Model file for the job. Use its own axes, mm. Face numbers are marked on the shaded views. A direction names the side the tool comes from. Coordinates: 2 decimals unless noted, no trailing zeros. Order: outer loops, then holes, each group sorted by start corner. A loop starts at its lowest first (then second) coordinate and runs counter-clockwise, first axis right, second up.
from build123d import *

# Parameters (mm, degrees)
SKETCH1_W           = 237.666601654
SKETCH1_H           = 144.870829151
BOSS_EXTRUDE1_DEPTH = 6.35
SKETCH6_R           = 4.7625
CUT_EXTRUDE1_DEPTH  = 279.412092375
BOSS_EXTRUDE2_DEPTH = 31.75
SKETCH8_R           = 3.5814
CUT_EXTRUDE2_DEPTH  = 165.026783357
FILLET1_R           = 3.81


with BuildPart() as part:
    # Sketch1 → Boss-Extrude1 (new body)
    with BuildSketch(Plane.XY):
        with Locations((118.833300827, 72.435414576)):
            Rectangle(SKETCH1_W, SKETCH1_H)
    extrude(amount=BOSS_EXTRUDE1_DEPTH)

    # Sketch6 → Cut-Extrude1 (cut, through all)
    with BuildSketch(Plane(origin=(0, 0, 0), x_dir=(-1, 0, 0), z_dir=(0, 0, -1))):
        with Locations((-216.35760516, 91.973324775)):
            Circle(SKETCH6_R)
        with Locations(Location((-118.912497493, 20.833508274, 0), (0, 0, 180))):
            Circle(SKETCH6_R)
        with BuildLine():
            Line((-237.666601654, 102.132216913), (-216.358133389, 102.133324761))
            ThreePointArc((-216.358133389, 102.133324761), (-208.163913134, 97.980737777), (-206.668218378, 88.91695703))
            Line((-206.668218378, 88.91695703), (-209.863652574, 78.786697699))
            ThreePointArc((-209.863652574, 78.786697699), (-210.516155402, 72.927274811), (-208.895904566, 67.258643251))
            Line((-208.895904566, 67.258643251), (-194.461394125, 39.056254914))
            ThreePointArc((-194.461394125, 39.056254914), (-186.82764399, 30.114000126), (-175.984822796, 25.567431049))
            Line((-175.984822796, 25.567431049), (-144.725556293, 20.41107019))
            ThreePointArc((-144.725556293, 20.41107019), (-138.832778099, 20.5948137), (-133.450682209, 23.001396414))
            Line((-133.450682209, 23.001396414), (-124.775487304, 29.13115556))
            ThreePointArc((-124.775487304, 29.13115556), (-114.240366099, 29.855525136), (-108.752497493, 20.833508274))
            Line((-108.752497493, 20.833508274), (-108.752497493, 0))
            Line((-108.752497493, 0), (33.78855799, -29.414686869))
            Line((33.78855799, -29.414686869), (48.645656143, 190.527142522))
            Line((48.645656143, 190.527142522), (-347.111633803, 192.661310616))
            Line((-347.111633803, 192.661310616), (-237.666601654, 102.132216913))
        make_face()
    extrude(amount=-CUT_EXTRUDE1_DEPTH, mode=Mode.SUBTRACT)

    # Sketch7 → Boss-Extrude2 (add)
    with BuildSketch(Plane.XY.offset(6.35)):
        Polygon((231.316601654, 102.132547055), (237.666601654, 102.132216913), (237.666601654, 0), (231.316601654, 0), align=None)
    extrude(amount=BOSS_EXTRUDE2_DEPTH)

    # Sketch8 → Cut-Extrude2 (cut, through all)
    with BuildSketch(Plane.ZY.offset(-231.316601654)):
        with Locations((23.289062999, 76.03064494)):
            Circle(SKETCH8_R)
        with Locations((23.289062999, 28.982263142)):
            Circle(SKETCH8_R)
    extrude(amount=-CUT_EXTRUDE2_DEPTH, mode=Mode.SUBTRACT)

    # Fillet1
    fillet1_edges = [part.edges().sort_by_distance(p)[0] for p in [
        (108.752497493, 0, 3.175),
        (231.316601654, 51.066273528, 6.35),
        (234.491601654, 0, 38.1),
        (234.491601654, 102.132381984, 38.1),
    ]]
    fillet(fillet1_edges, radius=FILLET1_R)


solid = part.part
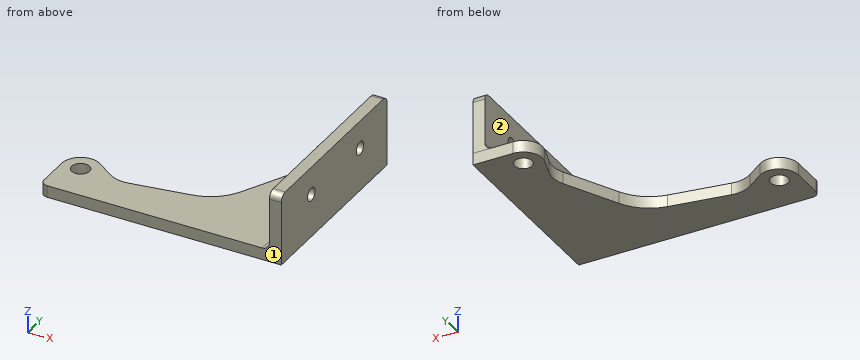
Q1. Cut at A-A, the plane x = 219. List the corners of the cut face in (y, z), plus the area to 3 significant figures.
Established:
outline: (0, 0) - (88.01, 0) - (88.01, 6.35) - (0, 6.35) - close; (95.94, 0) - (102.13, 0) - (102.13, 6.35) - (95.94, 6.35) - close
area: 598 mm2
Q2. Cut at C-C, the plane y = 84.5. List the corners of the cut face in (x, z), plus the area to 3 significant figures.
Established:
outline: (208.06, 0) - (237.67, 0) - (237.67, 38.1) - (231.32, 38.1) - (231.32, 10.16) arc R3.81 cw to (227.51, 6.35) - (208.06, 6.35) - close
area: 393 mm2
Q3. Cut at B-B, the plane z = 3.5. List the corners of the cut face in (x, y) (1 decimal).
Established:
outline: (108.8, 3.8) arc R3.8 ccw to (112.6, 0) - (237.7, 0) - (237.7, 102.1) - (216.4, 102.1) arc R10.2 ccw to (206.7, 88.9) - (209.9, 78.8) arc R15.2 cw to (208.9, 67.3) - (194.5, 39.1) arc R25.4 cw to (176, 25.6) - (144.7, 20.4) arc R15.2 cw to (133.5, 23) - (124.8, 29.1) arc R10.2 ccw to (108.8, 20.8) - close; hole circle Ø9.5 at (118.9, 20.8); hole circle Ø9.5 at (216.4, 92)
Q4. Cut at D-D, the plane x = 119. List the corners of the cut face in (y, z).
Established:
outline: (0, 0) - (16.07, 0) - (16.07, 6.35) - (0, 6.35) - close; (25.6, 0) - (30.99, 0) - (30.99, 6.35) - (25.6, 6.35) - close
Q5. Probe line 1 (X direction, y = 24.5, z = 23); line 2 (Z direction, x = 227.5, y = 67); line 3 (Z direction, x = 229.5, y = 68). List the from-to ranges inside material, lowest first.
Established:
line 1: x = 231.32 to 237.67
line 2: z = 0 to 6.35
line 3: z = 0 to 6.91
Q6. Drop flat-ended pins along their axis: P1, Ø8, axis at y = 28.98, z = 23.29, coming from the -X side; P2, Ø11, axis at x = 216.36, y = 91.97, coming from the +Z side. Give the stop position or say it passes through.
Established:
P1: stops at x = 231.32
P2: stops at z = 6.35
Q7. Which spindle directions (+Z, -Z, +X, -X, +Y, -Y) get a long thin tool onto all of the face, cutting with end or side? Do the marked faces 1 and 2. Say none if no direction does.
Established:
face 1: +Z, -Z, +X, -X, -Y
face 2: +Z, -X, +Y, -Y
